```python
from build123d import *

# Parameters (mm, degrees)
BOSS_EXTRUDE1_START = -46.439051
BOSS_EXTRUDE1_DEPTH = 61.439051
SKETCH2_W           = 24
SKETCH2_H           = 11.5
BOSS_EXTRUDE2_DEPTH = 10
BOSS_EXTRUDE3_START = -24
BOSS_EXTRUDE3_DEPTH = 24
SKETCH4_R           = 2
CUT_EXTRUDE1_DEPTH  = 24
CUT_EXTRUDE2_START  = -73.272081
CUT_EXTRUDE2_DEPTH  = 73.272081


with BuildPart() as part:
    # Sketch1 → Boss-Extrude1 (new body)
    with BuildSketch(Plane.XY.offset(BOSS_EXTRUDE1_START)):
        with BuildLine():
            Line((-17.5, 16.5), (-22, 16.5))
            Line((-22, 16.5), (-22, 9.5))
            ThreePointArc((-22, 9.5), (-20.681980515, 6.318019485), (-17.5, 5))
            Line((-17.5, 5), (17.5, 5))
            ThreePointArc((17.5, 5), (20.681980515, 6.318019485), (22, 9.5))
            Line((22, 9.5), (22, 16.5))
            Line((22, 16.5), (-17.5, 16.5))
        make_face()
    extrude(amount=BOSS_EXTRUDE1_DEPTH)

    # Sketch2 → Boss-Extrude2 (add)
    with BuildSketch(Plane.XY.offset(15)):
        with Locations((0, 10.75)):
            Rectangle(SKETCH2_W, SKETCH2_H)
    extrude(amount=BOSS_EXTRUDE2_DEPTH)

    # Sketch3 → Boss-Extrude3 (add)
    with BuildSketch(Plane(origin=(12, 0, 0), x_dir=(0, 0, -1), z_dir=(1, 0, 0)).offset(BOSS_EXTRUDE3_START)):
        with BuildLine():
            Line((-25, 5), (-25, 16.5))
            ThreePointArc((-25, 16.5), (-30.75, 10.75), (-25, 5))
        make_face()
    extrude(amount=BOSS_EXTRUDE3_DEPTH)

    # Sketch4 → Cut-Extrude1 (cut)
    with BuildSketch(Plane(origin=(12, 0, 0), x_dir=(0, 0, -1), z_dir=(1, 0, 0))):
        with Locations(Location((-25, 10.75, 0), (0, 0, 90))):
            Circle(SKETCH4_R)
    extrude(amount=-CUT_EXTRUDE1_DEPTH, mode=Mode.SUBTRACT)

    # Sketch5 → Cut-Extrude2 (cut)
    with BuildSketch(Plane(origin=(0, 0, -46.439050788), x_dir=(-1, 0, 0), z_dir=(0, 0, -1)).offset(CUT_EXTRUDE2_START)):
        with BuildLine():
            Line((22, 16.5), (-22, 16.5))
            Line((-22, 16.5), (-22, 9.5))
            ThreePointArc((-22, 9.5), (-20.681980515, 6.318019485), (-17.5, 5))
            Line((-17.5, 5), (17.5, 5))
            ThreePointArc((17.5, 5), (20.681980515, 6.318019485), (22, 9.5))
            Line((22, 9.5), (22, 16.5))
        make_face()
        with BuildLine():
            Line((21.7, 16.2), (-21.7, 16.2))
            Line((-21.7, 16.2), (-21.7, 9.5))
            ThreePointArc((-21.7, 9.5), (-20.469848481, 6.530151519), (-17.5, 5.3))
            Line((-17.5, 5.3), (17.5, 5.3))
            ThreePointArc((17.5, 5.3), (20.469848481, 6.530151519), (21.7, 9.5))
            Line((21.7, 9.5), (21.7, 16.2))
        make_face(mode=Mode.SUBTRACT)
    extrude(amount=CUT_EXTRUDE2_DEPTH, mode=Mode.SUBTRACT)


solid = part.part
```
Design review of the part built by this model. Coordinates are the model's own, in mm. A direction names the side the tool comes from. Round coordinates to 2 decimals unless told otherwise and drop trailing zeros. Write each loop counter-clockwise with the first axis right and the second up, starting at its lowest first coordinate (ties: lowest second). Pieces come first, ordered by that corner, then holes. Notation, with made-up numbers: (-30, -21.75) -> (-25, -21.75) arc R15 ccw to (-25, 6.25) -> close; hole circle Ø5 at (87, 85.5). An arc over 180 degrees is marked (long way). Write item = value, one per line. Start each with the question number.
1) Wall thickness on probe 1 along Z at (x, y) = (18, 6.75); probe 2 along Z at (x, y) = (-7.5, 10.5); probe 3 along X at (y, z) = (9.25, -29.5): over which ranges is each line inside the solid? List them lowest first. Write a range as from..to.
2) Clearance check with flat-ended pins moving along their axes: pin 1 (3 mm diameter, centred on x = -15, y = 11.5, fed in from +Z); pin 2 (3.5 mm diameter, centred on y = 8, z = 22.5, fed in from +X); pin 3 (1.5 mm diameter, centred on y = 14, z = 18.5, fed in from -X). State where each tip first meets the part, or that it passes through.
3) Take a section at D-D, the plane z = -5. State the section outline as (x, y) points, plus the area to 3 significant figures.
4) Take a section at B-B, the plane y = 10.75. State the section outline as (x, z) points.
5) Take a section at C-C, the plane x = -6. State the section outline as (y, z) points.
6) Take a section at A-A, the plane z = 25. State the section outline as (x, y) points.
7) Tool access review of faces 1 (the face through (-12, 11, 21)), 2 (the face through (17, 11, 15)), 3 (the face through (21.7, 13, -15)): name each direction out of +Z, -Z, +X, -X, +Y, -Y from which nothing blocks a thin tool from reaching the whole face with its end or side.
8) Mouldability with a two-part tool opening along Y and no side actions: class faces 4 (the face through (0, 11, -46.439)), 5 (the face through (0, 5.3, -9)), 6 (the face through (-0.17, 10.85, 30.75)), 7 (the face through (0.168, 9.163, 23.783)) as +Y half, -Y half, draft (parallel to the pull), parting line (faces both ways), or undercut.
Results list:
q1.probe_1 = -46.44..15
q1.probe_2 = -46.44..23.02, 26.98..30.74
q1.probe_3 = -21.69..21.69
q2.pin_1 = 15
q2.pin_2 = 12
q2.pin_3 = -12
q3.outline = (-21.7, 9.5) arc R4.2 ccw to (-17.5, 5.3) -> (17.5, 5.3) arc R4.2 ccw to (21.7, 9.5) -> (21.7, 16.2) -> (-21.7, 16.2) -> close
q3.area = 465 mm²
q4.outline = (-21.7, -46.44) -> (21.7, -46.44) -> (21.7, 15) -> (12, 15) -> (12, 23) -> (-12, 23) -> (-12, 15) -> (-21.7, 15) -> close; (-12, 27) -> (12, 27) -> (12, 30.75) -> (-12, 30.75) -> close
q5.outline = (5.3, -46.44) -> (16.2, -46.44) -> (16.2, 26.83) arc R5.75 ccw to (5.3, 26.83) -> close; hole circle Ø4 at (10.75, 25)
q6.outline = (-12, 5.3) -> (12, 5.3) -> (12, 8.75) -> (-12, 8.75) -> close; (-12, 12.75) -> (12, 12.75) -> (12, 16.2) -> (-12, 16.2) -> close
q7.face_1 = +Z, -X, +Y, -Y
q7.face_2 = +Z, +X, +Y, -Y
q7.face_3 = +Z, -Z, +X, +Y, -Y
q8.face_4 = draft
q8.face_5 = -Y half
q8.face_6 = parting line
q8.face_7 = undercut
